Solid Edge part; units mm, degrees
sketch "Sketch1" plane through (0, 0, 0) normal (0, -1, 0) x (1, 0, 0)
  line L0 (200, 28) -> (0, 28)
  line L1 (0, 28) -> (0, 0)
  line L2 (0, 0) -> (200, 0)
  line L3 (200, 0) -> (200, 28)
extrude "Protrusion1" add sketch "Sketch1" against normal blind 4
sketch "Sketch2" plane through (77.37, 0, 14) normal (0, -1, 0) x (1, 0, 0)
  line L0 (102.63, -11) -> (-57.3035, -11)
  line L1 (-57.3035, -11) -> (-57.3035, -14)
  line L2 (-57.3035, -14) -> (102.63, -14)
  line L3 (102.63, -14) -> (102.63, -11)
extrude "Protrusão_Extrudada_6" add sketch "Sketch2" along normal blind 5
sketch "Sketch3" plane through (77.37, 0, 14) normal (0, -1, 0) x (1, 0, 0)
  line L0 (102.63, -11) -> (-57.3035, -11)
  line L1 (-57.3035, -11) -> (-57.3035, -14)
  line L2 (-57.3035, -14) -> (102.63, -14)
  line L3 (102.63, -14) -> (102.63, -11)
extrude "Protrusão_Extrudada_7" add sketch "Sketch3" against normal blind 19
sketch "Sketch4" plane through (77.37, 0, 14) normal (0, -1, 0) x (-1, 0, 0)
  line L0 (-102.63, -14) -> (-102.63, 11)
  line L1 (-102.63, 11) -> (-122.63, 11)
  line L2 (-122.63, 11) -> (-122.63, -14)
  line L3 (-122.63, -14) -> (-102.63, -14)
  line L4 (57.3035, -14) -> (57.3035, 11)
  line L5 (57.3035, 11) -> (77.37, 11)
  line L6 (77.37, 11) -> (77.37, -14)
  line L7 (77.37, -14) -> (57.3035, -14)
extrude "Recorte_Extrudado_5" cut sketch "Sketch4" against normal blind 2
sketch "Sketch5" plane through (77.37, 0, 14) normal (0, -1, 0) x (1, 0, 0)
  line L0 (102.63, -14) -> (102.63, -11)
  line L1 (102.63, -11) -> (122.63, -11)
  line L2 (122.63, -14) -> (122.63, -11)
  line L3 (102.63, -14) -> (122.63, -14)
extrude "Recorte_Extrudado_6" cut sketch "Sketch5" against normal blind 21.6353
sketch "Sketch6" plane through (0, 0, 0) normal (0, -1, 0) x (1, 0, 0)
  line L0 (20.0665, 3) -> (20.0665, 0)
  line L1 (0, 0) -> (20.0665, 0)
  line L2 (0, 3) -> (0, 0)
  line L3 (20.0665, 3) -> (0, 3)
extrude "Recorte_Extrudado_7" cut sketch "Sketch6" against normal blind 21.2624
The model under review builds one solid part; all positions refer to its coordinate system, in mm. A direction names the side the tool comes from. Round coordinates to 2 decimals unless told otherwise and drop trailing zeros. Loops run counter-clockwise (first coordinate to the right, second up) from the corner with the lowest first, then second, coordinate; pieces in that order, holes last. Notation, with made-up numbers: (54, 30) - (109, 30) arc R17 cw to (109, 51) - close; hole circle Ø4 at (84.25, 44.5). An arc over 180 degrees is marked (long way). Use a Markdown table: item, result. Add a question column.
Q1. Add section B-B (z = 21). State the section outline as (x, y) points, plus the area to 3 significant figures.
Q2. Add section D-D (x = 184). State the section outline as (y, z) points.
Q3. Machinability: for faces 1 (the face through (101, 0, 16)), 2 (the face through (10, 2, 15)), 3 (the face through (101, 2, 28)), 4 (the face through (101, 4, 16)), 5 (the face through (190, 2, 16)), which of the approach directions +Z, -Z, +X, -X, +Y, -Y give a long, thin tool a straight path to every point of the face, cutting with its end or side? Answer none if there is none.
Q4. For probe 1 along Z at (x, y) = (69, 13); probe 2 along X at (y, z) = (0.25, 25.25); probe 3 along Y at (x, z) = (109, 22.25), list the stretches that pass through material, from the lowest coordinate up.
Q5. Add section C-C (y = 17). State the section outline as (x, z) points, plus the area to 3 significant figures.
Q6. Add section A-A (x = 62). State the section outline as (y, z) points, plus the area to 3 significant figures.
Q7. Insertion check: pin 1 Ø2 at (y, z) = (2, 16.5) entering from -X; pin 2 Ø16 at (x, z) = (10, 16) entering from -Y; pin 3 Ø1.5 at (x, y) = (90.5, -3) entering from +Z; pin 4 Ø7.5 at (x, z) = (114.5, 15.5) entering from +Y. Each pin has a flat end and moves straight along its axis. Give the tip position at first contact, or say it passes through.
Worked answers:
| question | item | result |
|---|---|---|
| 1 | outline | (0, 2) - (20.07, 2) - (20.07, 0) - (180, 0) - (180, 2) - (200, 2) - (200, 4) - (0, 4) - close |
| 1 | area | 720 mm² |
| 2 | outline | (2, 3) - (4, 3) - (4, 28) - (2, 28) - close |
| 3 | face 1 | +Z, +X, -X, -Y |
| 3 | face 2 | +Z, -Z, -X, -Y |
| 3 | face 3 | +Z, +X, -X, +Y, -Y |
| 3 | face 4 | +Z, +X, -X, +Y |
| 3 | face 5 | +Z, -Z, +X, -Y |
| 4 | probe 1 | 0 to 3 |
| 4 | probe 2 | 20.07 to 180 |
| 4 | probe 3 | 0 to 4 |
| 5 | outline | (20.07, 0) - (180, 0) - (180, 3) - (20.07, 3) - close |
| 5 | area | 480 mm² |
| 6 | outline | (-5, 0) - (19, 0) - (19, 3) - (4, 3) - (4, 28) - (0, 28) - (0, 3) - (-5, 3) - close |
| 6 | area | 172 mm² |
| 7 | pin 1 | x = 0 |
| 7 | pin 2 | y = 2 |
| 7 | pin 3 | z = 3 |
| 7 | pin 4 | y = 4 |
